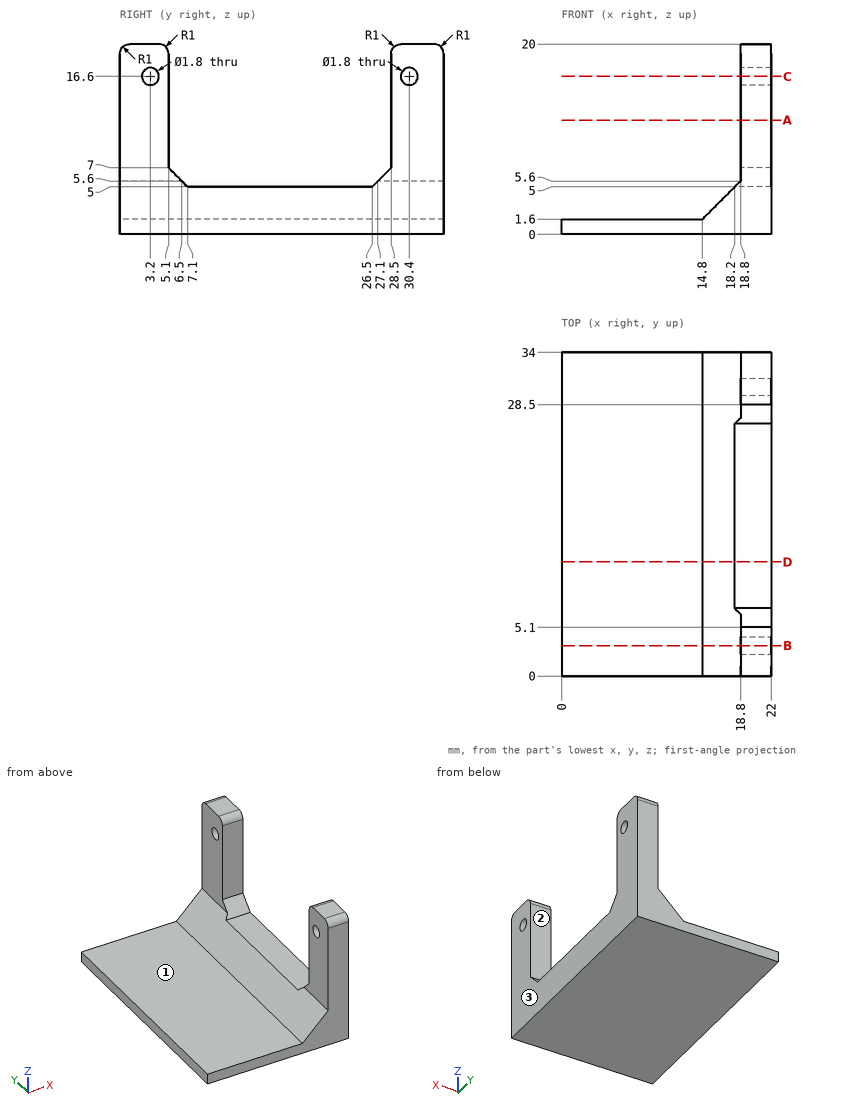
Answer from the drawing. Dimensions are ordinates in mm from the lowest x, y and z of the part. A direction names the side the tool comes from. Coordinates: 2 decimals unless noted, no trailing zeros. Write each loop counter-clockwise with the first axis right and the second up, starting at its lowest first coordinate (ties: lowest second). Pieces come first, ordered by that corner, then holes. Notation, with made-up numbers: (73, 75.5) - (77, 75.5) arc R34 ccw to (77, 112.5) - close; hole circle Ø6 at (3.25, -39). An arc over 180 degrees is marked (long way). One line per question, with ' | ' between items.
Q1. Find section A-A, the plane z = 12. Write down the section's boundary in (x, y).
Result set:
outline: (18.8, 0) - (22, 0) - (22, 5.1) - (18.8, 5.1) - close; (18.8, 28.5) - (22, 28.5) - (22, 34) - (18.8, 34) - close
Q2. Each of these flat-tipped pins is pushed along its axis until it touches: P1, Ø3.5, axis at y = 4.5, z = 16, coming from the -X side; P2, Ø1.9, axis at x = 20, y = 17, coming from the +Z side; P3, Ø5, axis at x = 12.5, y = 18, coming from the +Z side. Where does it stop, or does it pass through?
Result set:
P1: x = 18.8 | P2: z = 5 | P3: z = 1.8
Q3. Find section B-B, the plane y = 3.2. Write down the section's boundary in (x, z), plus the area to 3 significant figures.
Result set:
outline: (0, 0) - (22, 0) - (22, 15.7) - (18.8, 15.7) - (18.8, 5.6) - (14.8, 1.6) - (0, 1.6) - close; (18.8, 17.5) - (22, 17.5) - (22, 20) - (18.8, 20) - close | area: 96.3 mm^2
Q4. Consider L1, parallel to Y at x = 20.8, z = 16.6; L2, parallel to Z at x = 19.75, y = 30.4; L3, parallel to Y at x = 19.25, z = 12.5. Determine where each line is inside the solid, lowest interval first. Write a range as [from, to].
Result set:
L1: [0, 2.3], [4.1, 5.1], [28.5, 29.5], [31.3, 34] | L2: [0, 15.7], [17.5, 20] | L3: [0, 5.1], [28.5, 34]
Q5. For the marked faces 1, 2 and 3, determine the directions among +Z, -Z, +X, -X, +Y, -Y from which every point of the face is accessible in a straight line to the end or side of a thin tool.
Result set:
face 1: +Z, -X, +Y, -Y | face 2: +Z, +X, -X | face 3: +Z, -Z, +X, +Y, -Y
Q6. Find section D-D, the plane y = 12. Write down the section's boundary in (x, z).
Result set:
outline: (0, 0) - (22, 0) - (22, 5) - (18.2, 5) - (14.8, 1.6) - (0, 1.6) - close
Q7. Find section C-C, the plane z = 16.6. Write down the section's boundary in (x, y), plus the area to 3 significant figures.
Result set:
outline: (18.8, 0) - (22, 0) - (22, 2.3) - (18.8, 2.3) - close; (18.8, 4.1) - (22, 4.1) - (22, 5.1) - (18.8, 5.1) - close; (18.8, 28.5) - (22, 28.5) - (22, 29.5) - (18.8, 29.5) - close; (18.8, 31.3) - (22, 31.3) - (22, 34) - (18.8, 34) - close | area: 22.4 mm^2
